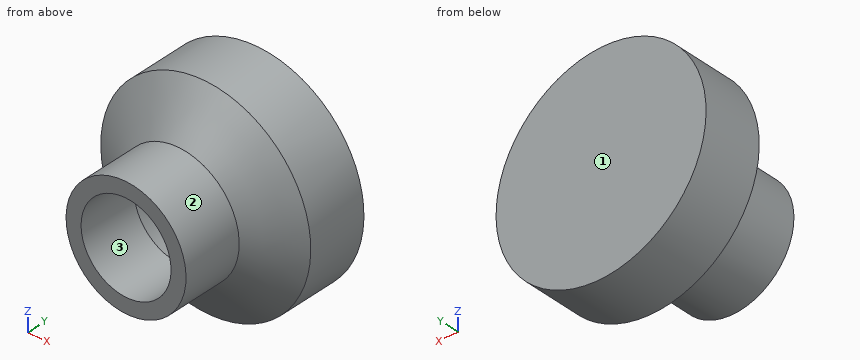
```python
from build123d import *

# Parameters (mm, degrees)
F3_D     = 6
F3_DEPTH = 4
F3_TIP   = 1.8025818571


with BuildPart() as f1:
    # F0 (on Right) → F1 (revolve)
    with BuildSketch(Plane.YZ):
        Polygon((-4, 4), (-4, 0), (6, 0), (6, 7), (2, 7), (0, 4), align=None)
    revolve(axis=Axis((0, 1, 0), (0, 1, 0)))

    # F3
    with Locations(Plane.XZ.offset(4)):
        with Locations((0, 0)):
            Hole(F3_D / 2, depth=F3_DEPTH)
            with Locations((0, 0, -(F3_DEPTH + F3_TIP / 2))):  # 118° drill point
                Cone(0, F3_D / 2, F3_TIP, mode=Mode.SUBTRACT)


solid = f1.part
```
Can you work these out from the model? Positions are in its coordinate system, mm. Face numbers are marked on the shaded views. Coordinates: 2 decimals unless noted, no trailing zeros. Loops run counter-clockwise (first coordinate to the right, second up) from the corner with the lowest first, then second, coordinate; pieces in that order, holes last. Notation, with made-up numbers: M -29.75,30 L -6.75,30 A19 cw -6.75,59 Z; hole C -8,34.5 d11. An arc over 180 degrees is marked long. Put each result on its own line as item: value. Start each with the question number.
(1) Imagine slicing it at A-A on y = 4. List the corners of the cut face in (x, z) for me.
(2) I need wall thicknesses on probe 1 along X at (y, z) = (-2.8, 0); probe 2 along Z at (x, y) = (-4.25, 4); probe 3 along Z at (x, y) = (0.25, 0.25). Which ranges of each line are inside material? Lowest first, please.
(3) We'd pull the mould along X, two halves only. Please class the marked faces 1, 2 and 3: +X half, -X half, draft (parallel to the pull), parting line (faces both ways), or undercut.
(4) Will these pins go through, and if not, where does the flat tip stop? pin 1 Ø3 at (y, z) = (3.5, 4) entering from -X; pin 2 Ø2 at (y, z) = (0.5, -4) entering from -X; pin 3 Ø6 at (y, z) = (-0.5, -2.5) entering from +X.
(5) Imagine slicing it at B-B on y = -0.5. List the corners of the cut face in (x, z) for me.
Worked answers:
1. outline: C 0,0 d14
2. probe 1: x = -4 to -3, 3 to 4
2. probe 2: z = -5.56 to 5.56
2. probe 3: z = -4.37 to -2.57, 2.57 to 4.37
3. face 1: draft
3. face 2: parting line
3. face 3: undercut
4. pin 1: stops at x = -6.54
4. pin 2: stops at x = -4.96
4. pin 3: stops at x = 6.95
5. outline: C 0,0 d8; hole C 0,0 d6
